Design review of the part built by this model. Coordinates are the model's own, in mm. Face numbers are marked on the shaded views. A direction names the side the tool comes from. Round coordinates to 2 decimals unless told otherwise and drop trailing zeros. Loops run counter-clockwise (first coordinate to the right, second up) from the corner with the lowest first, then second, coordinate; pieces in that order, holes last. Notation, with made-up numbers: M 68,1 L 83,1 A29 cw 83,28 Z; hole C 61,13 d2. An arc over 180 degrees is marked long. One line per item, written item: value. Start each with the question number.
Item 1: For the marked faces 4 and 5, list the 3-axis set-ups (+Z, -Z, +X, -X, +Y, -Y) from which the entire face can be reached by the end or side of a thin tool; tool diameter is ignored.
Item 2: Mouldability with a two-part tool opening along Y and no side actions: class the marked faces 1, 2 and 3 as released by +Y, released by -Y, zero draft, split by the parting line, or undercut.
Item 3: For line 1 along Y through (x, z) = (13, -12.25); line 2 along Y through (x, z) = (111, -15.25); line 3 along X through (y, z) = (-15.5, -9.75), list the stretches that pass through material, from the lowest coordinate up.
Item 4: We need section B-B (x = 31). Write out the cut boundary in (y, z).
Item 5: We need section A-A (z = -8.5). State how many separate pieces and enclosed holes the cut face has, then the cut area to 3 significant figures.
Item 6: Clearance check with flat-ended pins moving along their axes: pin 1 (4 mm diameter, centred on x = 84.5, y = -24, fed in from +Z); pin 2 (6 mm diameter, centred on x = 12, y = -13.5, fed in from +Z). State where each tip first meets the part, or that it passes through.
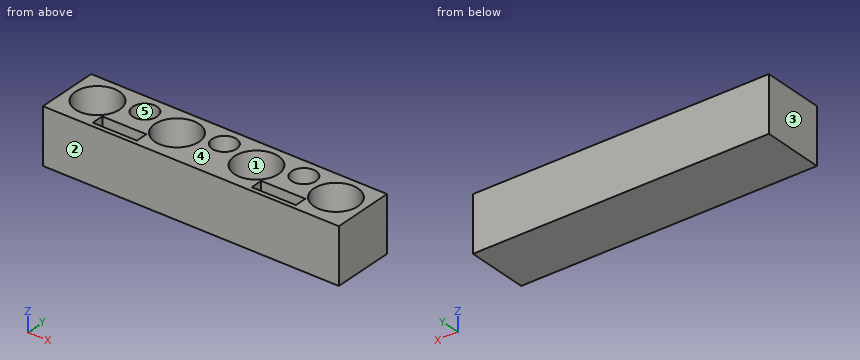
from build123d import *

# Parameters (mm, degrees)
F0_W     = 134.0499884313
F0_H     = 28
F0_W_2   = 20
F0_H_2   = 5
F0_R     = 10
F0_R_2   = 5.55
F1_DEPTH = 23
F3_START = 20.5
F3_DEPTH = 5.5
F4_W     = 134.0499884313
F4_H     = 2
F5_DEPTH = 28


with BuildPart() as f1:
    # F0 (on Top) → F1 (new body)
    with BuildSketch(Plane.XY):
        with Locations((67.0249942156, -14)):
            Rectangle(F0_W, F0_H)
        with Locations((31.0064340452, -23.5)):
            Rectangle(F0_W_2, F0_H_2, mode=Mode.SUBTRACT)
        with Locations((103.0416570261, -23.5)):
            Rectangle(F0_W_2, F0_H_2, mode=Mode.SUBTRACT)
        with Locations((13, -13)):
            Circle(F0_R, mode=Mode.SUBTRACT)
        with Locations((31.0083314052, -8.55)):
            Circle(F0_R_2, mode=Mode.SUBTRACT)
        with Locations((49.0166628104, -13)):
            Circle(F0_R, mode=Mode.SUBTRACT)
        with Locations((85.0333256209, -13)):
            Circle(F0_R, mode=Mode.SUBTRACT)
        with Locations((67.0249942156, -8.55)):
            Circle(F0_R_2, mode=Mode.SUBTRACT)
        with Locations((121.0499884313, -13)):
            Circle(F0_R, mode=Mode.SUBTRACT)
        with Locations((103.0416570261, -8.55)):
            Circle(F0_R_2, mode=Mode.SUBTRACT)
        with Locations((31.0064340452, -23.5)):
            Rectangle(F0_W_2, F0_H_2)
        with Locations((103.0416570261, -23.5)):
            Rectangle(F0_W_2, F0_H_2)
    extrude(amount=-F1_DEPTH)

    # F2 (on Front) → F3 (cut)
    with BuildSketch(Plane.XZ.offset(F3_START)):
        with BuildLine():
            Line((21.00643, -12), (41.00643, -12))
            ThreePointArc((41.00643, -12), (31.00643, -2), (21.00643, -12))
        make_face()
        with BuildLine():
            ThreePointArc((21.00643, -12), (31.00643, -22), (41.00643, -12))
            Line((41.00643, -12), (21.00643, -12))
        make_face()
        with BuildLine():
            ThreePointArc((21.00643, -12), (31.00643, -2), (41.00643, -12))
            Line((41.00643, -12), (41.00643, 6))
            Line((41.00643, 6), (21.00643, 6))
            Line((21.00643, 6), (21.00643, -12))
        make_face()
        with BuildLine():
            Line((93.04166, -12), (113.04166, -12))
            ThreePointArc((113.04166, -12), (103.04166, -2), (93.04166, -12))
        make_face()
        with BuildLine():
            ThreePointArc((93.04166, -12), (103.04166, -22), (113.04166, -12))
            Line((113.04166, -12), (93.04166, -12))
        make_face()
        with BuildLine():
            ThreePointArc((93.04166, -12), (103.04166, -2), (113.04166, -12))
            Line((113.04166, -12), (113.04166, 6))
            Line((113.04166, 6), (93.04166, 6))
            Line((93.04166, 6), (93.04166, -12))
        make_face()
    extrude(amount=F3_DEPTH, mode=Mode.SUBTRACT)

    # F4 (on Front) → F5 (join)
    with BuildSketch(Plane.XZ):
        with Locations((67.0249942156, -24)):
            Rectangle(F4_W, F4_H)
    extrude(amount=F5_DEPTH)


solid = f1.part
A:
1. face 4: +Z, +X, -X, +Y, -Y
1. face 5: +Z
2. face 1: undercut
2. face 2: released by -Y
2. face 3: zero draft
3. line 1: -28 to -23, -3 to 0
3. line 2: -28 to -26, -20.5 to 0
3. line 3: 0 to 3.32, 22.68 to 39.33, 58.7 to 75.35, 94.72 to 111.37, 130.73 to 134.05
4. outline: M -28,-25 L 0,-25 L 0,0 L -3,0 L -3,-23 L -14.1,-23 L -14.1,0 L -20.5,0 L -20.5,-22 L -26,-22 L -26,0 L -28,0 Z
5. separate pieces: 1
5. enclosed holes: 9
5. area: 1,990 mm2
6. pin 1: z = 0
6. pin 2: z = -23
